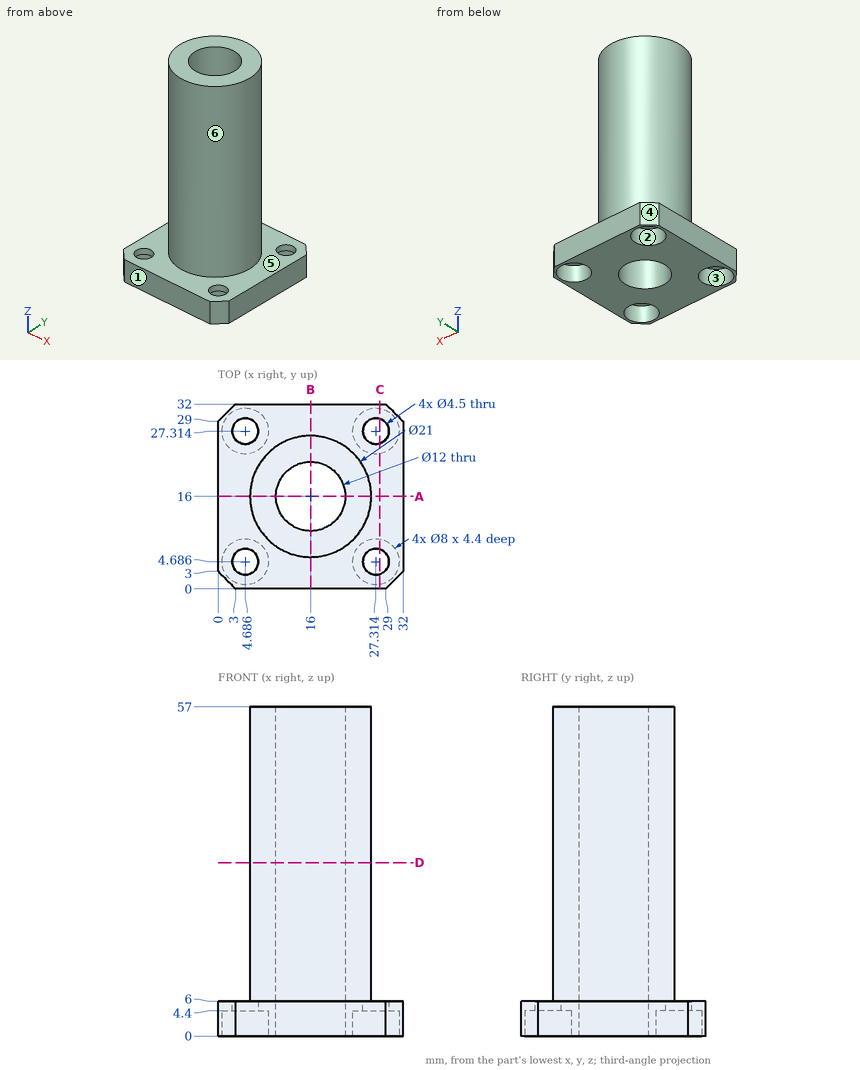
Geometry check sheet. Reference: drawing and pictorial views, mm from the part's lowest x, y, z. A direction names the side the tool comes from. Give positions to 0.01 mm unless a question says otherwise; leave off trailing zeros. Order: outer loops, then holes, each group sorted by start corner. A loop starts at its lowest first (then second) coordinate and runs counter-clockwise, first axis right, second up. Notation, with made-up numbers: M 17,77 L 29,77 A14 ccw 29,90 Z; hole C 73.5,18 d3. An arc over 180 degrees is marked long. Return JSON: item names as keys, results as strings. Group by question number.
1) Access from +Z, -Z, +X, -X, +Y, -Y to the whole of each face (thin tool, end or side, straight path). Record for the marked faces 1 and 2.
2) Section check A-A on y = 16. Record the cut outline in (x, z), and give its area (3 significant figures).
3) Mould release check, pull along X, two halves, no side actions. Record for the marked faces 3, 4, 5 and 6: pulls with the +X half, pulls with the -X half, needs draft (parallel to the pull), parting line crosses it, or undercut.
4) Section check C-C on x = 28. Record the cut outline in (y, z).
5) Scan lines: line 1 (X direction, y = 5, z = 5) (1 decimal); line 2 (X direction, y = 15.5, z = 10); line 3 (X direction, y = 19, z = 6.5) (1 decimal). Record each from-to range of solid material in increasing order.
6) Section check D-D on z = 30. Record the cut outline in (x, y).
7) Go/stop test with flat-tipped pins: pin 1 Ø1 at (y, z) = (8, 38.5) entering from +X; pin 2 Ø3 at (x, z) = (16, 41.5) entering from +Y; pin 3 Ø4 at (x, y) = (5.5, 29) entering from -Z. Record where each tip stops, or that it passes through.
Answer block:
{
 "1": {"face 1": "+Z, -Z, +X, -X, -Y", "face 2": "-Z"},
 "2": {"outline": "M 0,0 L 10,0 L 10,57 L 5.5,57 L 5.5,6 L 0,6 Z; M 22,0 L 32,0 L 32,6 L 26.5,6 L 26.5,57 L 22,57 Z", "area": "579 mm^2"},
 "3": {"face 3": "undercut", "face 4": "pulls with the -X half", "face 5": "needs draft", "face 6": "parting line crosses it"},
 "4": {"outline": "M 0,0 L 0.75,0 L 0.75,4.4 L 2.54,4.4 L 2.54,6 L 0,6 Z; M 6.83,4.4 L 8.63,4.4 L 8.63,0 L 23.37,0 L 23.37,4.4 L 25.17,4.4 L 25.17,6 L 6.83,6 Z; M 29.46,4.4 L 31.25,4.4 L 31.25,0 L 32,0 L 32,6 L 29.46,6 Z"},
 "5": {"line 1": "x = 0 to 2.5, 6.9 to 25.1, 29.5 to 32", "line 2": "x = 5.51 to 10.02, 21.98 to 26.49", "line 3": "x = 5.9 to 10.8, 21.2 to 26.1"},
 "6": {"outline": "C 16,16 d21; hole C 16,16 d12"},
 "7": {"pin 1": "stops at x = 23.35", "pin 2": "stops at y = 26.5", "pin 3": "stops at z = 4.4"}
}
